Can you work these out from the drawing? Everything is in mm from the part's minimum corner. Give positions to 0.01 mm unless a question says otherwise; leave off trailing zeros. Loops run counter-clockwise (first coordinate to the right, second up) from the corner with the lowest first, then second, coordinate; pieces in that order, holes last. Notation, with made-up numbers: (14.5, -39.75) -> (34.5, -39.75) arc R38 ccw to (34.5, -0.75) -> close; hole circle Ø7 at (38.5, 49.25). An arc over 180 degrees is marked (long way). Write item = value, one per line. Start each with the question number.
1) If we mould it in two halves opening along Y, with no side actions, what happens to the marked faces 1, 2 and 3? For each: +Y half, -Y half, draft (parallel to the pull), parting line (faces both ways), or undercut.
2) I want a section at C-C (x = 25.4). Count the separate pieces of the cut face and the enclosed holes in it, and give its area (3 significant figures).
3) I want a section at B-B (z = 2). List the corners of the cut face in (x, y) for me, and give its area (3 significant figures).
4) I'm going to push flat-ended pins straight in: pin 1 Ø6.5 at (x, y) = (25.4, 12.7) entering from +Z; pin 2 Ø4 at (x, y) = (25.4, 69.85) entering from -Z; pin 3 Ø7.5 at (x, y) = (25.4, 25.4) entering from +Z. Where does each tip first touch, or does it pass through?
5) I need wall thicknesses on probe 1 along X at (y, z) = (24, 5); probe 2 along Y at (x, z) = (4, 4.75); probe 3 along X at (y, z) = (37, 5.5). Which ranges of each line are inside material? Lowest first, please. Write a range as from..to.
6) I want a section at A-A (y = 38.1). List the corners of the cut face in (x, z) for me, and give its area (3 significant figures).
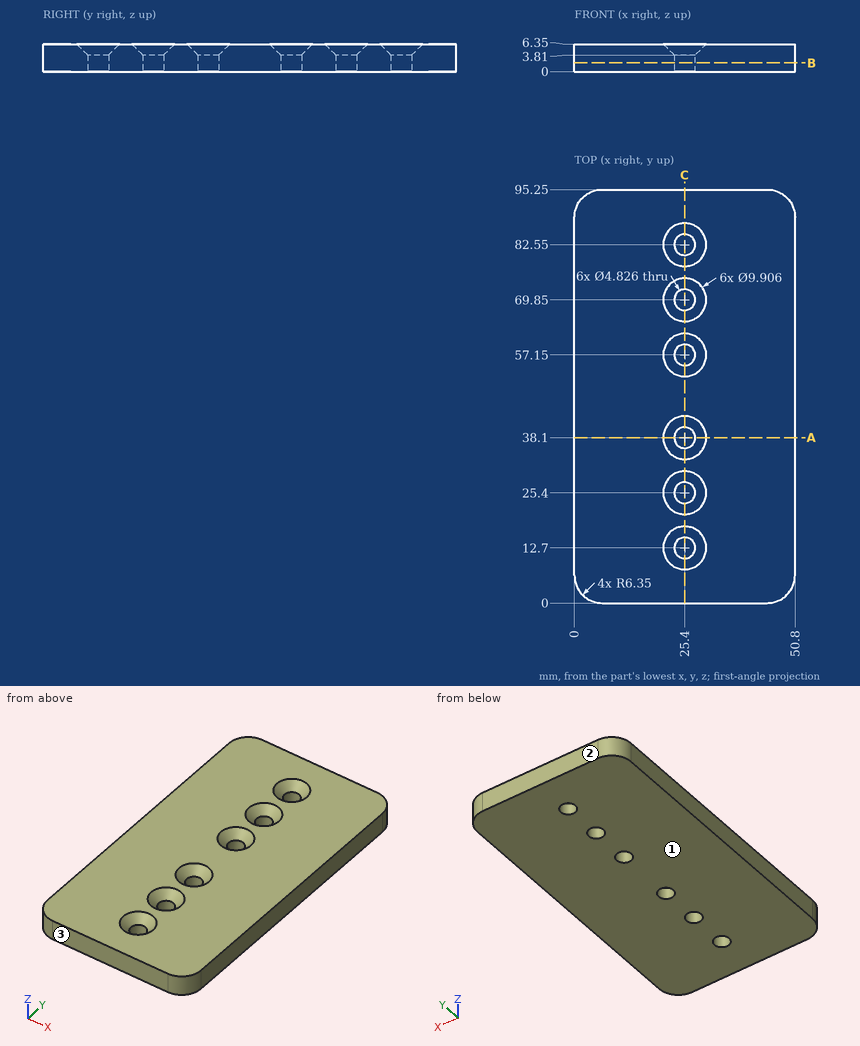
Answer list:
q1.face_1 = draft
q1.face_2 = +Y half
q1.face_3 = -Y half
q2.separate_pieces = 7
q2.enclosed_holes = 0
q2.area = 382 mm^2
q3.outline = (0, 6.35) arc R6.35 ccw to (6.35, 0) -> (44.45, 0) arc R6.35 ccw to (50.8, 6.35) -> (50.8, 88.9) arc R6.35 ccw to (44.45, 95.25) -> (6.35, 95.25) arc R6.35 ccw to (0, 88.9) -> close; hole circle Ø4.83 at (25.4, 12.7); hole circle Ø4.83 at (25.4, 25.4); hole circle Ø4.83 at (25.4, 38.1); hole circle Ø4.83 at (25.4, 57.15); hole circle Ø4.83 at (25.4, 69.85); hole circle Ø4.83 at (25.4, 82.55)
q3.area = 4,690 mm^2
q4.pin_1 = 4.65
q4.pin_2 = through
q4.pin_3 = 5.15
q5.probe_1 = 0..22.08, 28.72..50.8
q5.probe_2 = 0.45..94.8
q5.probe_3 = 0..21.45, 29.35..50.8
q6.outline = (0, 0) -> (22.99, 0) -> (22.99, 3.81) -> (20.45, 6.35) -> (0, 6.35) -> close; (27.81, 0) -> (50.8, 0) -> (50.8, 6.35) -> (30.35, 6.35) -> (27.81, 3.81) -> close
q6.area = 285 mm^2
